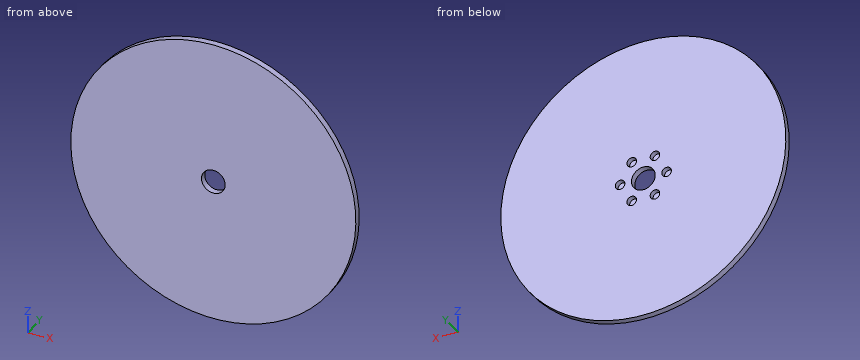
from build123d import *

# Parameters (mm, degrees)
SKETCH1_R             = 90
BOSS_EXTRUDE1_DEPTH   = 4
SKETCH2_R             = 7.5
CUT_EXTRUDE1_DEPTH    = 128.342059038
SKETCH3_R             = 3.023767703
CUT_EXTRUDE2_DEPTH    = 3.297006
CIRPATTERN1_START     = 0.702994223
CIRPATTERN1_OUTLINE_R = 3.023767703
CIRPATTERN1_DEPTH     = 3.297005777


# Read off the part's stored shape, not the designer's step: CirPattern1
with BuildPart() as part:
    # Sketch1 → Boss-Extrude1 (new body)
    with BuildSketch(Plane(origin=(0, 0, 0), x_dir=(1, 0, 0), z_dir=(0, 1, 0))):
        with Locations(Location((0, 0, 0), (0, 0, 270))):
            Circle(SKETCH1_R)
    extrude(amount=BOSS_EXTRUDE1_DEPTH)

    # Sketch2 → Cut-Extrude1 (cut, through all)
    with BuildSketch(Plane(origin=(0, 0, 0), x_dir=(1, 0, 0), z_dir=(0, 1, 0))):
        with Locations(Location((0, 0, 0), (0, 0, 270))):
            Circle(SKETCH2_R)
    extrude(amount=CUT_EXTRUDE1_DEPTH, mode=Mode.SUBTRACT)

    # Sketch3 → Cut-Extrude2 (cut)
    with BuildSketch(Plane(origin=(0, 4, 0), x_dir=(1, 0, 0), z_dir=(0, 1, 0))):
        with Locations(Location((-14.689580211, 0, 0), (0, 0, 270))):
            Circle(SKETCH3_R)
    extrude(amount=-CUT_EXTRUDE2_DEPTH, mode=Mode.SUBTRACT)

    # CirPattern1 outline → CirPattern1 (cut)
    with BuildSketch(Plane(origin=(0, 0, 0), x_dir=(1, 0, 0), z_dir=(0, 1, 0)).offset(CIRPATTERN1_START)):
        with Locations((-7.344790105, -12.721549634)):
            Circle(CIRPATTERN1_OUTLINE_R)
        with Locations((7.344790105, -12.721549634)):
            Circle(CIRPATTERN1_OUTLINE_R)
        with Locations((14.689580211, 0)):
            Circle(CIRPATTERN1_OUTLINE_R)
        with Locations((7.344790105, 12.721549634)):
            Circle(CIRPATTERN1_OUTLINE_R)
        with Locations((-7.344790105, 12.721549634)):
            Circle(CIRPATTERN1_OUTLINE_R)
    extrude(amount=CIRPATTERN1_DEPTH, mode=Mode.SUBTRACT)


solid = part.part
Verification items for the finished model (mm, model axes). Coordinates: 2 decimals unless noted, no trailing zeros. Order: outer loops, then holes, each group sorted by start corner. A loop starts at its lowest first (then second) coordinate and runs counter-clockwise, first axis right, second up. Notation, with made-up numbers: M 4.5,55 L 28.5,55 A14 cw 28.5,81 Z; hole C 89,9.5 d1. An arc over 180 degrees is marked long. One line per item, written item: value. Start each with the question number.
Item 1: Depth check by flat-ended pin: P1, Ø9, axis at x = 0, z = 0, coming from the +Y side; P2, Ø1.8, axis at x = -7.5, z = -11.5, coming from the +Y side; P3, Ø2, axis at x = 2, y = 1, coming from the +Z side; P4, Ø2, axis at y = 2, z = 35, coming from the +X side. Enter the tip coordinate at first touch or a pass-through.
Item 2: Sectioned sample at C-C on y = 1.75. Record the cut outline in (x, z).
Item 3: Sectioned sample at B-B on z = 0. Record the cut outline in (x, y), then the cut area to 3 significant figures.
Item 4: Sectioned sample at D-D on x = 27. Record the cut outline in (y, z), then the cut area to 3 significant figures.
Item 5: Thickness scan on probe 1 along X at (y, z) = (2.8, 0); probe 2 along X at (y, z) = (1.2, 2); probe 3 along Z at (x, y) = (-1, 2.3). Record the ranges inside material, lowest first.
Item 6: Sectioned sample at A-A on x = 0. Record the cut outline in (y, z).
Calculated:
1. P1: through
1. P2: y = 0.7
1. P3: z = 89.99
1. P4: x = 83.33
2. outline: C 0,0 d180; hole C -14.69,0 d6.05; hole C -7.34,-12.72 d6.05; hole C -7.34,12.72 d6.05; hole C 0,0 d15; hole C 7.34,-12.72 d6.05; hole C 7.34,12.72 d6.05; hole C 14.69,0 d6.05
3. outline: M -90,0 L -7.5,0 L -7.5,4 L -11.67,4 L -11.67,0.7 L -17.71,0.7 L -17.71,4 L -90,4 Z; M 7.5,0 L 90,0 L 90,4 L 17.71,4 L 17.71,0.7 L 11.67,0.7 L 11.67,4 L 7.5,4 Z
3. area: 620 mm^2
4. outline: M 0,-85.85 L 4,-85.85 L 4,85.85 L 0,85.85 Z
4. area: 687 mm^2
5. probe 1: -90 to -17.71, -11.67 to -7.5, 7.5 to 11.67, 17.71 to 90
5. probe 2: -89.98 to -16.96, -12.42 to -7.23, 7.23 to 12.42, 16.96 to 89.98
5. probe 3: -89.99 to -7.43, 7.43 to 89.99
6. outline: M 0,-90 L 4,-90 L 4,-7.5 L 0,-7.5 Z; M 0,7.5 L 4,7.5 L 4,90 L 0,90 Z
